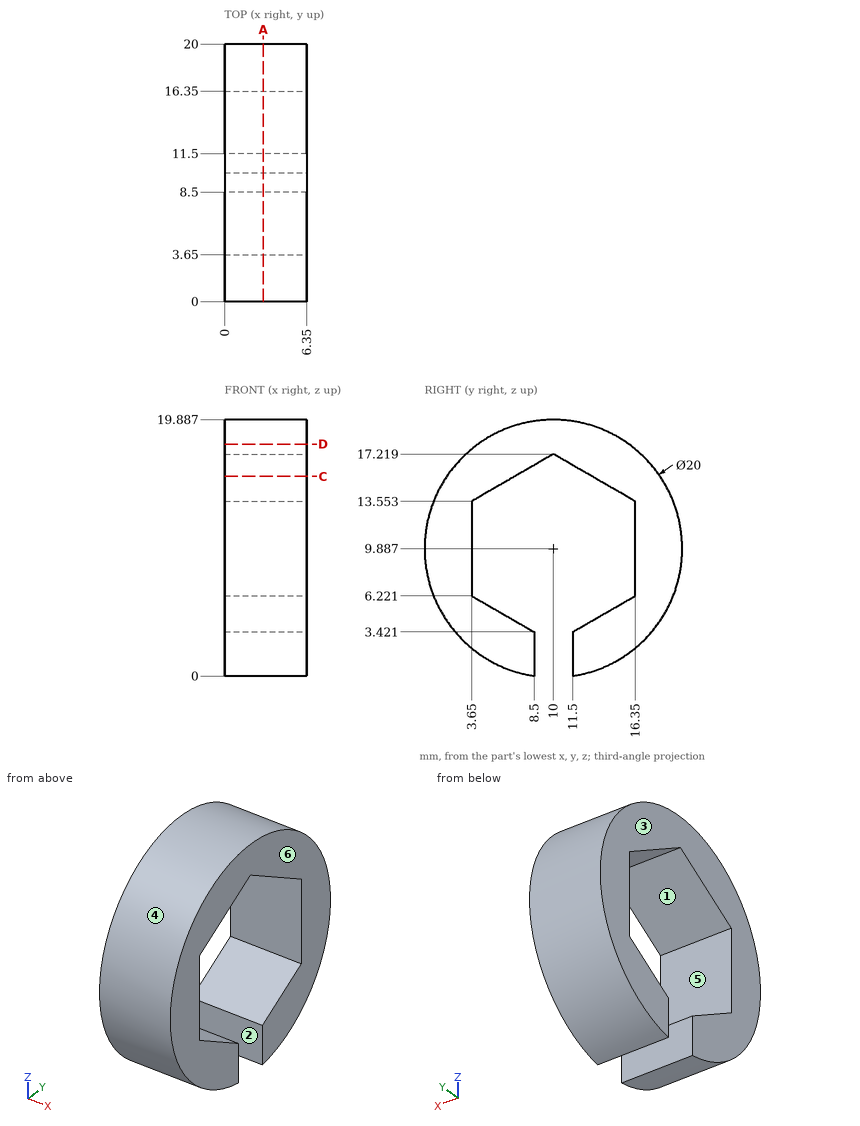
Job drawing, mm, ordinate dimensions from the low corner. One solid piece. A direction names the side the tool comes from. Coordinates: 2 decimals unless noted, no trailing zeros. Write each loop counter-clockwise with the first axis right and the second up, starting at its lowest first coordinate (ties: lowest second). Pieces come first, ordered by that corner, then holes.
Item 1: Slice it at D-D (z = 18). Write the cut outline in (x, y).
Item 2: Which spindle directions (+Z, -Z, +X, -X, +Y, -Y) get a long thin tool onto all of the face, cutting with end or side? Do the marked faces 1, 2 and 3. Say none if no direction does.
Item 3: Slice it at C-C (z = 15.5). Write the cut outline in (x, y).
Item 4: Slice it at A-A (x = 3). Write the cut outline in (y, z), and give its area (3 significant figures).
Item 5: Probe line 1 (Y direction, x = 4.5, z = 10); line 2 (Z direction, x = 4.75, y = 13.75) (1 decimal); line 3 (Z direction, x = 2.5, y = 4) (1 decimal). List the from-to ranges inside material, lowest first.
Item 6: Pin check, flat tips, straight feed: pin 1 (3 mm diameter, centred on x = 3.5, y = 13, fed in from -Z); pin 2 (3 mm diameter, centred on x = 3.5, z = 15, fed in from +Y) (1 decimal); pin 3 (1 mm diameter, centred on y = 5.5, z = 6, fed in from +X); pin 4 (2 mm diameter, centred on x = 5, y = 4, fed in from -Z). Stop position of each tip, or through.
Item 7: Mould opens along Z. For the marked faces 4, 5 and 6 say: released by +Z, released by -Z, zero draft, split by the parting line, or undercut.
Results found:
1. outline: (0, 4.15) - (6.35, 4.15) - (6.35, 15.85) - (0, 15.85) - close
2. face 1: +X, -X
2. face 2: -Z, +X, -X
2. face 3: +Z, -Z, -X, +Y, -Y
3. outline: (0, 1.72) - (6.35, 1.72) - (6.35, 7.02) - (0, 7.02) - close; (0, 12.98) - (6.35, 12.98) - (6.35, 18.28) - (0, 18.28) - close
4. outline: (3.65, 6.22) - (3.65, 13.55) - (10, 17.22) - (16.35, 13.55) - (16.35, 6.22) - (11.5, 3.42) - (11.5, 0) arc R10 ccw (long way) to (8.5, 0) - (8.5, 3.42) - close
4. area: 165 mm2
5. line 1: y = 0 to 3.65, 16.35 to 20
5. line 2: z = 0.6 to 4.7, 15.1 to 19.2
5. line 3: z = 1.9 to 6, 13.8 to 17.9
6. pin 1: stops at z = 0
6. pin 2: stops at y = 19.3
6. pin 3: passes through
6. pin 4: stops at z = 1.23
7. face 4: split by the parting line
7. face 5: undercut
7. face 6: zero draft
